For this review, use the dimensioned drawing (mm, ordinates from the lowest corner) and the shaded views. Round coordinates to 2 decimals unless told otherwise and drop trailing zeros. Order: outer loops, then holes, each group sorted by start corner. A loop starts at its lowest first (then second) coordinate and runs counter-clockwise, first axis right, second up. Notation, with made-up numbers: (-22.5, -8.5) - (19.5, -8.5) arc R21 cw to (19.5, 11.5) - close; hole circle Ø1 at (53.5, 54). An arc over 180 degrees is marked (long way). Write each question's results on one line, items separated by ' | '. Start each with the question number.
(1) Take a section at A-A, the plane z = 3.9. Give the boundary of the cut face in (x, y), plus the area to 3 significant figures.
(2) Draft analysis for pull direction Z (two halves, no side actions). For the marked faces 1, 2 and 3, state which applies: pulls with the +Z half, pulls with the -Z half, needs draft (parallel to the pull), parting line crosses it, or undercut.
(3) For L1, parallel to Y at x = 4.5, z = 3.6; L2, parallel to Y at x = 3.65, z = 2.9; L3, parallel to Z at x = 4.35, y = 2.15, list the stretches that pass through material, from the lowest coordinate up. Write a range as from..to.
(4) Insertion check: pin 1 Ø0.9 at (y, z) = (1.5, 4.5) entering from -X; pin 2 Ø1.5 at (x, z) = (2, 2.5) entering from +Y. Each pin has a flat end and moves straight along its axis. Give the tip position at first contact, or say it passes through.
(5) Take a section at B-B, the plane y = 2.75. Give the boundary of the cut face in (x, z).
(6) Take a section at D-D, the plane y = 3.4. Give the boundary of the cut face in (x, z).
(7) Take a section at C-C, the plane x = 4.25. Give the boundary of the cut face in (y, z).
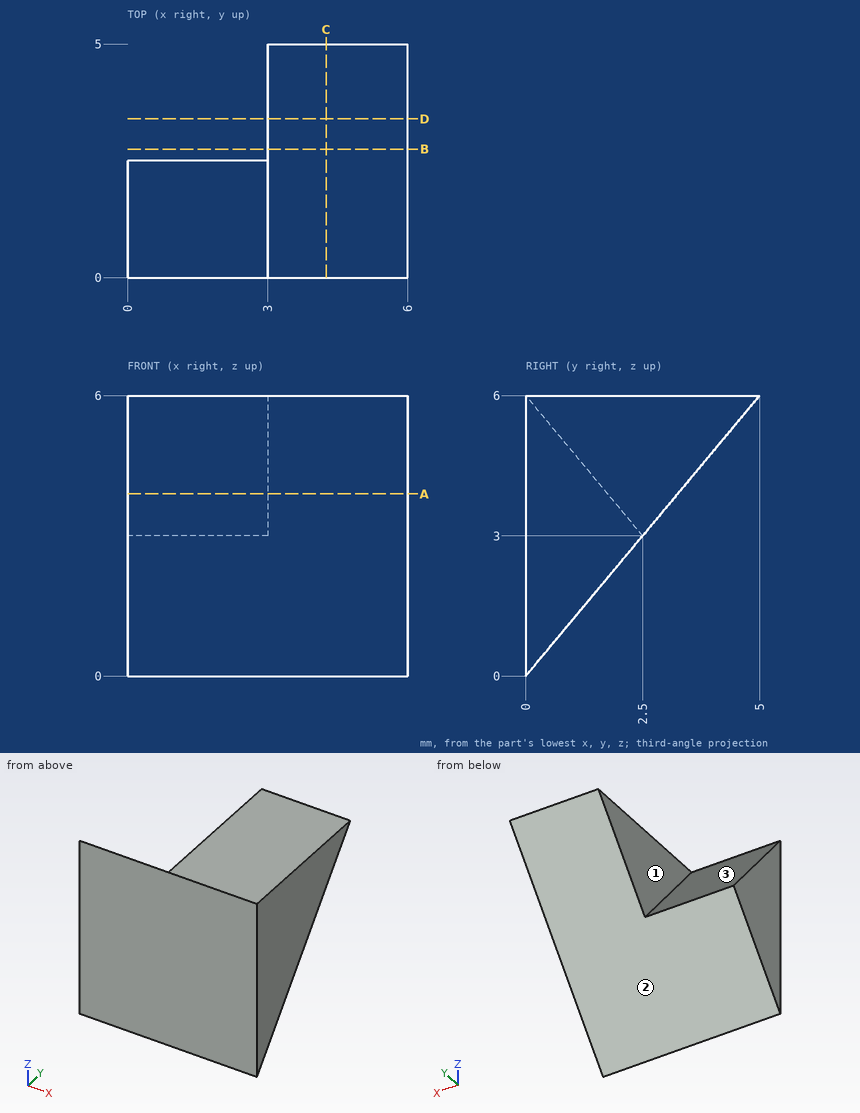
Results below:
1) outline: (0, 0) - (6, 0) - (6, 3.25) - (3, 3.25) - (3, 1.75) - (0, 1.75) - close | area: 15.0 mm^2
2) face 1: needs draft | face 2: pulls with the -Z half | face 3: pulls with the +Z half
3) L1: y = 0..3 | L2: y = 0..2.42 | L3: z = 2.58..6
4) pin 1: stops at x = 0 | pin 2: stops at y = 2.5
5) outline: (3, 3.3) - (6, 3.3) - (6, 6) - (3, 6) - close
6) outline: (3, 4.08) - (6, 4.08) - (6, 6) - (3, 6) - close
7) outline: (0, 0) - (5, 6) - (0, 6) - close
